Verification items for the finished model (mm, model axes). Face numbers are marked on the shaded views. A direction names the side the tool comes from. Coordinates: 2 decimals unless noted, no trailing zeros. Write each loop counter-clockwise with the first axis right and the second up, starting at its lowest first coordinate (ties: lowest second). Pieces come first, ordered by that corner, then holes. Notation, with made-up numbers: (8, 43) -> (60, 43) arc R19 cw to (60, 75) -> close; hole circle Ø6 at (32.25, 77.25). An arc over 180 degrees is marked (long way). Write item = value, one per line. Start each with the question number.
(1) Section check B-B (x = 19.5). Record the cut outline in (y, z).
(2) Material ranges on probe 1 along X at (y, z) = (47, -16.5); probe 2 along Z at (x, y) = (-16, 60.5); probe 3 along X at (y, z) = (69, -21.5), recorded low to high. Write a range as [from, to].
(3) Set-up check for the marked faces 1, 2, 3 and 4: record each of +Z, -Z, +X, -X, +Y, -Y from which the full face is reachable in a straight line by a thin tool's end or side.
(4) Gauge pin test, flat ends, axial feed: pin 1 Ø15 at (x, y) = (-14.5, 53) entering from +Z; pin 2 Ø24 at (y, z) = (69.5, -33) entering from +X; pin 3 Ø6 at (x, y) = (13.5, 70.5) entering from -Z. Record the tip position at first contact, or that the pin passes through.
(5) Section check A-A (y = 30). Record the cut outline in (x, z), plus the area to 3 significant figures.
(6) Section check D-D (y = 70). Record the cut outline in (x, z).
(7) Section check C-C (z = -5). Record the cut outline in (x, y).
```python
from build123d import *

# Parameters (mm, degrees)
SKETCH1_W           = 30
SKETCH1_H           = 80
BOSS_EXTRUDE1_DEPTH = 50
BOSS_EXTRUDE2_DEPTH = 15
BOSS_EXTRUDE3_DEPTH = 20
SKETCH2_W           = 25
SKETCH2_H           = 45
BOSS_EXTRUDE4_DEPTH = 30
SKETCH3_W           = 75
SKETCH3_H           = 25
BOSS_EXTRUDE7_DEPTH = 65
SKETCH7_W           = 75
SKETCH7_H           = 20
BOSS_EXTRUDE8_DEPTH = 30
CUT_EXTRUDE6_DEPTH  = 144.614066163
CUT_EXTRUDE7_DEPTH  = 75
SKETCH11_W          = 5
SKETCH11_H          = 35
BOSS_EXTRUDE9_DEPTH = 30


with BuildPart() as part:
    # Sketch1 → Boss-Extrude1 (new body)
    with BuildSketch(Plane.XY):
        with Locations((-15, 40)):
            Rectangle(SKETCH1_W, SKETCH1_H)
    extrude(amount=-BOSS_EXTRUDE1_DEPTH)



with BuildPart() as body_2:
    # Sketch1_3 → Boss-Extrude2 (new body)
    with BuildSketch(Plane.XY):
        Polygon((100, 0), (0, 0), (0, 80), (25, 80), (25, 20), (100, 20), align=None)
    extrude(amount=BOSS_EXTRUDE2_DEPTH)


with BuildPart() as part_1:
    add(part.part)

    add(body_2.part)  # Boss-Extrude3 merges body 2
    # Sketch1_4 → Boss-Extrude3 (add)
    with BuildSketch(Plane.XY):
        Polygon((100, 0), (0, 0), (0, 80), (25, 80), (25, 20), (100, 20), align=None)
    extrude(amount=-BOSS_EXTRUDE3_DEPTH)

    # Sketch2 → Boss-Extrude4 (add)
    with BuildSketch(Plane(origin=(0, 0, -20), x_dir=(-1, 0, 0), z_dir=(0, 0, -1))):
        with Locations((-12.5, 22.5)):
            Rectangle(SKETCH2_W, SKETCH2_H)
    extrude(amount=BOSS_EXTRUDE4_DEPTH)

    # Sketch3 → Boss-Extrude7 (add)
    with BuildSketch(Plane.XY.offset(15)):
        with Locations((62.5, 32.5)):
            Rectangle(SKETCH3_W, SKETCH3_H)
    extrude(amount=-BOSS_EXTRUDE7_DEPTH)

    # Sketch7 → Boss-Extrude8 (add)
    with BuildSketch(Plane(origin=(0, 0, -20), x_dir=(-1, 0, 0), z_dir=(0, 0, -1))):
        with Locations((-62.5, 10)):
            Rectangle(SKETCH7_W, SKETCH7_H)
    extrude(amount=BOSS_EXTRUDE8_DEPTH)

    # Sketch8 → Cut-Extrude6 (cut, through all)
    with BuildSketch(Plane.XY.offset(15)):
        Polygon((100, 45), (100, 20), (45, 45), align=None)
    extrude(amount=-CUT_EXTRUDE6_DEPTH, mode=Mode.SUBTRACT)

    # Sketch9 → Cut-Extrude7 (cut)
    with BuildSketch(Plane(origin=(100, 0, 0), x_dir=(0, 0, -1), z_dir=(1, 0, 0))):
        Polygon((-15, 45), (20, 45), (-15, 20), align=None)
    extrude(amount=-CUT_EXTRUDE7_DEPTH, mode=Mode.SUBTRACT)

    # Sketch11 → Boss-Extrude9 (add)
    with BuildSketch(Plane(origin=(0, 0, -20), x_dir=(-1, 0, 0), z_dir=(0, 0, -1))):
        with Locations((-2.5, 62.5)):
            Rectangle(SKETCH11_W, SKETCH11_H)
    extrude(amount=BOSS_EXTRUDE9_DEPTH)


solid = part_1.part
```
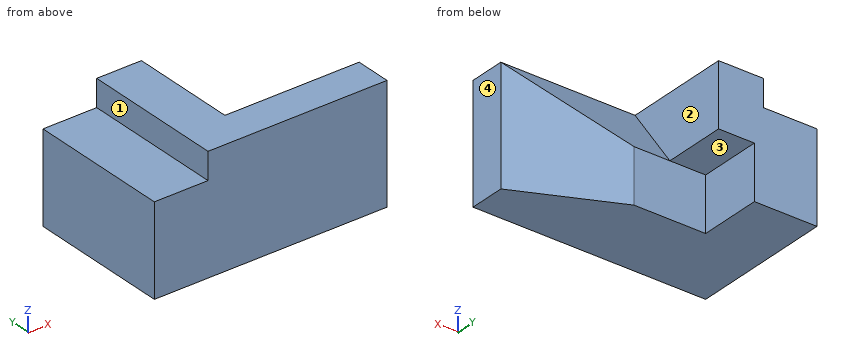
Response:
q1.outline = (0, -50) -> (45, -50) -> (45, -20) -> (80, -20) -> (80, 15) -> (0, 15) -> close
q2.probe_1 = [-30, 25]
q2.probe_2 = [-50, 0]
q2.probe_3 = [-30, 5]
q3.face_1 = +Z, -X, +Y, -Y
q3.face_2 = +Z, +X, +Y
q3.face_3 = -Z, +X, +Y
q3.face_4 = +Z, -Z, +X, +Y, -Y
q4.pin_1 = 0
q4.pin_2 = 5
q4.pin_3 = -20
q5.outline = (-30, -50) -> (78, -50) -> (78, 1) -> (25, 1) -> (25, 15) -> (0, 15) -> (0, 0) -> (-30, 0) -> close
q5.area = 5,830 mm2
q6.outline = (-30, -50) -> (5, -50) -> (5, -20) -> (25, -20) -> (25, 15) -> (0, 15) -> (0, 0) -> (-30, 0) -> close
q7.outline = (-30, 0) -> (100, 0) -> (100, 20) -> (68.57, 34.29) -> (25, 34.29) -> (25, 80) -> (-30, 80) -> close
